```python
from build123d import *

# Parameters (mm, degrees)
EXTRUDE_1_DEPTH     = 57.7
EXTRUDE_2_DEPTH     = 30.8
SKETCH_5_R          = 4
CUT_EXTRUDE_1_DEPTH = 15
SKETCH_7_W          = 6
SKETCH_7_H          = 7
SKETCH_7_R          = 2
EXTRUDE_3_DEPTH     = 2
SKETCH_8_W          = 6
SKETCH_8_H          = 1.5
EXTRUDE_4_DEPTH     = 6
EXTRUDE_START       = -37
SKETCH_8_3_W        = 6
SKETCH_8_3_H        = 1.5
EXTRUDE_5_DEPTH     = 6
SKETCH_9_R          = 2
CUT_EXTRUDE_2_DEPTH = 6
CUT_EXTRUDE_START   = -26.9
CUT_EXTRUDE_3_DEPTH = 26.9
CUT_EXTRUDE_4_DEPTH = 49.696406438
SKETCH_12_W         = 6
SKETCH_12_H         = 6
CUT_EXTRUDE_5_DEPTH = 10


with BuildPart() as part:
    # 스케치1 → 보스-돌출1 (new body)
    with BuildSketch(Plane.XY):
        with BuildLine():
            Line((-13.5, 0), (-18.5, 0))
            Line((-18.5, 0), (-18.5, -18.5))
            Line((-18.5, -18.5), (18.5, -18.5))
            Line((18.5, -18.5), (18.5, 0))
            Line((18.5, 0), (13.5, 0))
            ThreePointArc((13.5, 0), (0, -13.5), (-13.5, 0))
        make_face()
    extrude(amount=-EXTRUDE_1_DEPTH)

    # 스케치3 → 보스-돌출2 (add)
    with BuildSketch(Plane.XY.offset(-26.9)):
        with BuildLine():
            Line((-13.5, 0), (-11.5, 0))
            ThreePointArc((-11.5, 0), (0, -11.5), (11.5, 0))
            Line((11.5, 0), (13.5, 0))
            ThreePointArc((13.5, 0), (0, -13.5), (-13.5, 0))
        make_face()
    extrude(amount=-EXTRUDE_2_DEPTH)

    # 스케치5 → 컷-돌출1 (cut)
    with BuildSketch(Plane.ZY.offset(-18.5)):
        with Locations((-21.9, 0)):
            Circle(SKETCH_5_R)
    extrude(amount=CUT_EXTRUDE_1_DEPTH, mode=Mode.SUBTRACT)

    # 스케치7 → 보스-돌출3 (add)
    # profile 1 of 2: a face of its own
    with BuildSketch(Plane.XZ.offset(18.5)):
        with Locations((9.5, 3.5)):
            Rectangle(SKETCH_7_W, SKETCH_7_H)
        with Locations(Location((9.5, 4.15, 0), (0, 0, 270))):
            Circle(SKETCH_7_R, mode=Mode.SUBTRACT)
    # profile 2 of 2: a face of its own
    with BuildSketch(Plane.XZ.offset(18.5)):
        with Locations((-9.5, 3.5)):
            Rectangle(SKETCH_7_W, SKETCH_7_H)
        with Locations(Location((-9.5, 4.15, 0), (0, 0, 270))):
            Circle(SKETCH_7_R, mode=Mode.SUBTRACT)
    extrude_3 = extrude(amount=-EXTRUDE_3_DEPTH)

    # 대칭 복사1: 보스-돌출3 across plane
    add(extrude_3.mirror(Plane.XY.offset(-28.85)))

    # 스케치8 → 보스-돌출4 (add)
    with BuildSketch(Plane.ZY.offset(18.5)):
        with Locations((-5, -0.75)):
            Rectangle(SKETCH_8_W, SKETCH_8_H)
        with Locations((-52.7, -0.75)):
            Rectangle(SKETCH_8_W, SKETCH_8_H)
    extrude(amount=EXTRUDE_4_DEPTH)

    # 스케치8<3> → 보스-돌출5 (add)
    with BuildSketch(Plane.ZY.offset(18.5).offset(EXTRUDE_START)):
        with Locations((-5, -0.75)):
            Rectangle(SKETCH_8_3_W, SKETCH_8_3_H)
        with Locations((-52.7, -0.75)):
            Rectangle(SKETCH_8_3_W, SKETCH_8_3_H)
    extrude(amount=-EXTRUDE_5_DEPTH)

    # 스케치9 → 컷-돌출2 (cut)
    with BuildSketch(Plane(origin=(0, 0, 0), x_dir=(1, 0, 0), z_dir=(0, 1, 0))):
        with Locations(Location((-21.5, 52.7, 0), (0, 0, 180))):
            Circle(SKETCH_9_R)
        with Locations(Location((-21.5, 5, 0), (0, 0, 180))):
            Circle(SKETCH_9_R)
        with Locations(Location((21.5, 5, 0), (0, 0, 270))):
            Circle(SKETCH_9_R)
        with Locations(Location((21.5, 52.7, 0), (0, 0, 90))):
            Circle(SKETCH_9_R)
    extrude(amount=-CUT_EXTRUDE_2_DEPTH, mode=Mode.SUBTRACT)

    # 스케치10 → 컷-돌출3 (cut)
    with BuildSketch(Plane.XY.offset(CUT_EXTRUDE_START)):
        with BuildLine():
            Line((-13.5, 0), (-13.75, 0))
            ThreePointArc((-13.75, 0), (0, -13.75), (13.75, 0))
            Line((13.75, 0), (13.5, 0))
            ThreePointArc((13.5, 0), (0, -13.5), (-13.5, 0))
        make_face()
    extrude(amount=CUT_EXTRUDE_3_DEPTH, mode=Mode.SUBTRACT)

    # 스케치11 → 컷-돌출4 (cut, through all)
    with BuildSketch(Plane.XY.offset(-26.9)):
        with BuildLine():
            ThreePointArc((11.5, 0), (0, -11.5), (-11.5, 0))
            Line((-11.5, 0), (-12.5, 0))
            ThreePointArc((-12.5, 0), (0, -12.5), (12.5, 0))
            Line((12.5, 0), (11.5, 0))
        make_face()
    extrude(amount=-CUT_EXTRUDE_4_DEPTH, mode=Mode.SUBTRACT)

    # 스케치12 → 컷-돌출5 (cut)
    with BuildSketch(Plane(origin=(0, 0, 0), x_dir=(1, 0, 0), z_dir=(0, 1, 0))):
        with Locations((-21.5, 5)):
            Rectangle(SKETCH_12_W, SKETCH_12_H)
    extrude(amount=-CUT_EXTRUDE_5_DEPTH, mode=Mode.SUBTRACT)


solid = part.part
```
Source: CAD feature listing. Evaluate the final solid. Frame: model axes, mm. A direction names the side the tool comes from. Give positions to 0.01 mm unless a question says otherwise; leave off trailing zeros. Loops run counter-clockwise (first coordinate to the right, second up) from the corner with the lowest first, then second, coordinate; pieces in that order, holes last. Notation, with made-up numbers: (65.25, 83.25) - (105.25, 83.25) arc R18 cw to (105.25, 96.25) - close; hole circle Ø6 at (-36, -17). An arc over 180 degrees is marked (long way). Use CSV: the item, a comma, the result in double quotes.
1) Cut plane D-D (z = -1). Output: boundary loops of the cut face in (x, y), and give its area (3 significant figures).
Worked out:
outline,"(-18.5, -18.5) - (18.5, -18.5) - (18.5, 0) - (13.75, 0) arc R13.75 cw to (-13.75, 0) - (-18.5, 0) - close"
area,"388 mm^2"
2) Pin query (flat end, axial travel): P1, Ø1.6, axis at y = -17.5, z = 3, coming from the +X side; P2, Ø0.6, axis at y = -17.5, z = 4.5, coming from the -X side; P3, Ø11, axis at x = 4, y = -6.5, coming from the +Z side. Return the tip coordinate at first contact, or that it passes through.
Worked out:
P1,"stops at x = 12.5"
P2,"stops at x = -12.5"
P3,"stops at z = -26.9"
3) Cut plane A-A (z = -61.85). Output: boundary loops of the cut face in (x, y), and give its area (3 significant figures).
Worked out:
outline,"(-12.5, -18.5) - (-11.5, -18.5) - (-11.5, -16.5) - (-12.5, -16.5) - close; (-7.5, -18.5) - (-6.5, -18.5) - (-6.5, -16.5) - (-7.5, -16.5) - close; (6.5, -18.5) - (7.5, -18.5) - (7.5, -16.5) - (6.5, -16.5) - close; (11.5, -18.5) - (12.5, -18.5) - (12.5, -16.5) - (11.5, -16.5) - close"
area,"8.00 mm^2"
4) Cut plane C-C (y = -6.25). Output: boundary loops of the cut face in (x, z), and give its area (3 significant figures).
Worked out:
outline,"(-18.5, -57.7) - (-10.83, -57.7) - (-10.83, -26.9) - (-12.25, -26.9) - (-12.25, 0) - (-18.5, 0) - close; (10.83, -57.7) - (18.5, -57.7) - (18.5, 0) - (12.25, 0) - (12.25, -26.9) - (10.83, -26.9) - close"
area,"809 mm^2"
5) Set-up query: faces 1 (the flat face through (21, -1, -8)), 2 (the flat face through (-12.5, -18, 3)), 3 (the flat face through (-9.54, -16.5, -59.69)). Return all of +Z, -Z, +X, -X, +Y, -Y with unobstructed straight access to the full face (end or side cutting, diameter ignored); none if empty.
Worked out:
face 1,"+X, +Y, -Y"
face 2,"+Z, -X, +Y, -Y"
face 3,"-Z, +X, -X, +Y"
6) Line query: line 1 (X direction, y = -17.2, z = 4.15); line 2 (X direction, y = -0.9, z = -5); line 3 (X direction, y = -16.75, z = -32). Output: solid intervals per line, ascending.
Worked out:
line 1,"x = -12.5 to -11.5, -7.5 to -6.5, 6.5 to 7.5, 11.5 to 12.5"
line 2,"x = -18.5 to -13.72, 13.72 to 19.5, 23.5 to 24.5"
line 3,"x = -18.5 to 18.5"
7) Cut plane B-B (x = -21.5). Output: boundary loops of the cut face in (y, z).
Worked out:
outline,"(-1.5, -55.7) - (0, -55.7) - (0, -54.7) - (-1.5, -54.7) - close; (-1.5, -50.7) - (0, -50.7) - (0, -49.7) - (-1.5, -49.7) - close"
